Source: CAD feature listing. Evaluate the final solid. Frame: model axes, mm. Give positions to 0.01 mm unless a question says otherwise; leave off trailing zeros. Order: outer loops, then holes, each group sorted by start corner. A loop starts at its lowest first (then second) coordinate and runs counter-clockwise, first axis right, second up.
1) Section A-A, the plane y = -90. Return loops of the section in (x, z), plus the area to 3 significant figures.
2) Section C-C, the plane y = 0. Return loops of the section in (x, z).
3) Section B-B, the plane x = -72. Return loops of the section in (y, z), plus the area to 3 significant figures.
4) First-contact query: P1, Ø6, axis at x = -6, y = 5.5, coming from the +Z side; P2, Ø23, axis at x = -2, y = -90, coming from the -Z side. Flat tips, straight axial feed; report the tip coordinate or a pass-through.
5) Material intervals for line 1 (Y direction, x = 68, z = 13.6); line 2 (X direction, y = -103, z = 6.5); line 3 (Y direction, x = -29, z = 4), sorted ascending.
6) Section D-D, the plane x = 68. Return loops of the section in (y, z), plus the area to 3 significant figures.
```python
from build123d import *

# Parameters (mm, degrees)
SKETCH_1_W               = 236
SKETCH_1_H               = 336
EXTRUDE_1_DEPTH          = 15
SHELL_2_T                = -2
SKETCH_2_W               = 232
SKETCH_2_H               = 332
SKETCH_2_W_2             = 216
SKETCH_2_H_2             = 316
EXTRUDE_2_DEPTH          = 2
CUT_EXTRUDE_1_DEPTH      = 357.433724555
CUT_EXTRUDE_1_DEPTH_BACK = 357.433724555
SKETCH_3_R               = 1
SKETCH_4_R               = 20
SKETCH_4_R_2             = 10
CUT_EXTRUDE_2_DEPTH      = 2


with BuildPart() as part:
    # 草图1 → 凸台-拉伸1 (new body)
    with BuildSketch(Plane.XY):
        Rectangle(SKETCH_1_W, SKETCH_1_H)
    extrude(amount=EXTRUDE_1_DEPTH)

    # 抽壳2
    shell_2_openings = [part.faces().sort_by_distance(p)[0] for p in [
        (0, 0, 0),
    ]]
    offset(amount=SHELL_2_T, openings=shell_2_openings, kind=Kind.INTERSECTION)

    # 草图2 → 凸台-拉伸2 (add)
    with BuildSketch(Plane.XY):
        Rectangle(SKETCH_2_W, SKETCH_2_H)
        Rectangle(SKETCH_2_W_2, SKETCH_2_H_2, mode=Mode.SUBTRACT)
    extrude(amount=EXTRUDE_2_DEPTH)

    # 草图3 → 切除-拉伸1 (cut, two sides: drawn at the far end of the back side and taken through both)
    with BuildSketch(Plane(origin=(0, 168, 0), x_dir=(1, 0, 0), z_dir=(0, 1, 0)).offset(-CUT_EXTRUDE_1_DEPTH_BACK)):
        with Locations(Location((115, -12, 0), (0, 0, 270))):
            Circle(SKETCH_3_R)
    extrude(amount=CUT_EXTRUDE_1_DEPTH + CUT_EXTRUDE_1_DEPTH_BACK, mode=Mode.SUBTRACT)

    # 草图4 → 切除-拉伸2 (cut)
    with BuildSketch(Plane.XY.offset(15)):
        with Locations((-72, 0)):
            Circle(SKETCH_4_R)
        with Locations((-2, 0)):
            Circle(SKETCH_4_R_2)
        with Locations((68, 0)):
            Circle(SKETCH_4_R_2)
        with Locations((68, 90)):
            Circle(SKETCH_4_R_2)
        with Locations((-2, 90)):
            Circle(SKETCH_4_R_2)
        with Locations((68, -90)):
            Circle(SKETCH_4_R_2)
        with Locations((-2, -90)):
            Circle(SKETCH_4_R_2)
    extrude(amount=-CUT_EXTRUDE_2_DEPTH, mode=Mode.SUBTRACT)


solid = part.part
```
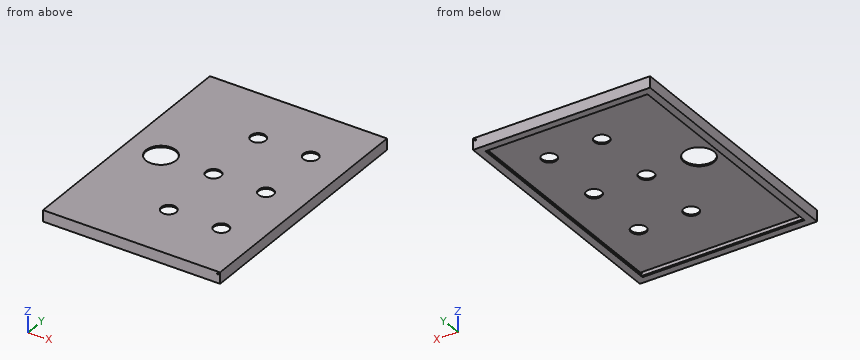
From the geometry:
1. outline: (-118, 0) - (-108, 0) - (-108, 2) - (-116, 2) - (-116, 13) - (-12, 13) - (-12, 15) - (-118, 15) - close; (8, 13) - (58, 13) - (58, 15) - (8, 15) - close; (78, 13) - (116, 13) - (116, 2) - (108, 2) - (108, 0) - (118, 0) - (118, 15) - (78, 15) - close
1. area: 476 mm2
2. outline: (-118, 0) - (-108, 0) - (-108, 2) - (-116, 2) - (-116, 13) - (-92, 13) - (-92, 15) - (-118, 15) - close; (-52, 13) - (-12, 13) - (-12, 15) - (-52, 15) - close; (8, 13) - (58, 13) - (58, 15) - (8, 15) - close; (78, 13) - (116, 13) - (116, 2) - (108, 2) - (108, 0) - (118, 0) - (118, 15) - (78, 15) - close
3. outline: (-168, 0) - (-158, 0) - (-158, 2) - (-166, 2) - (-166, 13) - (-20, 13) - (-20, 15) - (-168, 15) - close; (20, 13) - (166, 13) - (166, 2) - (158, 2) - (158, 0) - (168, 0) - (168, 15) - (20, 15) - close
3. area: 676 mm2
4. P1: passes through
4. P2: stops at z = 13
5. line 1: y = -168 to -100, -80 to -10, 10 to 80, 100 to 168
5. line 2: x = -118 to -116, 116 to 118
5. line 3: y = -168 to -166, 166 to 168
6. outline: (-168, 0) - (-158, 0) - (-158, 2) - (-166, 2) - (-166, 13) - (-100, 13) - (-100, 15) - (-168, 15) - close; (-80, 13) - (-10, 13) - (-10, 15) - (-80, 15) - close; (10, 13) - (80, 13) - (80, 15) - (10, 15) - close; (100, 13) - (166, 13) - (166, 2) - (158, 2) - (158, 0) - (168, 0) - (168, 15) - (100, 15) - close
6. area: 636 mm2
